from build123d import *

# Parameters (mm, degrees)
SALIENTE_EXTRUIR1_START                = 8
CROQUIS1_R                             = 10
SALIENTE_EXTRUIR1_DEPTH                = 258
CROQUIS2_R                             = 15
SALIENTE_EXTRUIR2_DEPTH                = 3
CORTAR_EXTRUIR1_REACH                  = 268.845
CORTAR_EXTRUIR1_END_RADIUS             = 10
CROQUIS3_R                             = 3.075
CORTAR_EXTRUIR1_DIRECTION_2_REACH      = 268.845
CORTAR_EXTRUIR1_DIRECTION_2_END_RADIUS = 10
CORTAR_EXTRUIR2_START                  = 10
CORTAR_EXTRUIR2_DEPTH                  = 3.5
TALADRO_ROSCADO_M61_D                  = 5
TALADRO_ROSCADO_M61_DEPTH              = 11.497848452
TALADRO_ROSCADO_M61_TIP                = 1.502151548
CORTAR_EXTRUIR3_START                  = 10
CORTAR_EXTRUIR3_DEPTH                  = 3.5
CORTAR_EXTRUIR4_START                  = 125.5
CROQUIS9_R                             = 10
CROQUIS9_R_2                           = 9.5
CORTAR_EXTRUIR4_DEPTH                  = 1.3
CORTAR_EXTRUIR5_START                  = 214.543146
CROQUIS10_R                            = 10
CROQUIS10_R_2                          = 9.5
CORTAR_EXTRUIR5_DEPTH                  = 1.3
CORTAR_EXTRUIR6_START                  = -8
CROQUIS11_R                            = 10
CROQUIS11_R_2                          = 9.5
CORTAR_EXTRUIR6_DEPTH                  = 1.3


with BuildPart() as part:
    # Croquis1 → Saliente-Extruir1 (new body)
    with BuildSketch(Plane(origin=(0, 0, 0), x_dir=(0, 0, -1), z_dir=(1, 0, 0)).offset(SALIENTE_EXTRUIR1_START)):
        Circle(CROQUIS1_R)
    extrude(amount=SALIENTE_EXTRUIR1_DEPTH)

    # Croquis2 → Saliente-Extruir2 (add)
    with BuildSketch(Plane.ZY.offset(-70.5)):
        Circle(CROQUIS2_R)
    extrude(amount=SALIENTE_EXTRUIR2_DEPTH)

    # Cortar-Extruir1: up to this cylinder (the profile starts inside it)
    cortar_extruir1_end = Plane(origin=(248.5, 0, 0), z_dir=(-1, 0, 0)) * Cylinder(CORTAR_EXTRUIR1_END_RADIUS, 558.69, mode=Mode.PRIVATE)
    # Croquis3 → Cortar-Extruir1 (cut, up to the surface)
    with BuildSketch(Plane.XY, mode=Mode.PRIVATE) as cortar_extruir1_sk1:
        with Locations((248.5, 0)):
            Circle(CROQUIS3_R)
    cortar_extruir1_tool1 = extrude(cortar_extruir1_sk1.sketch, amount=-CORTAR_EXTRUIR1_REACH, mode=Mode.PRIVATE) & cortar_extruir1_end
    add(cortar_extruir1_tool1.solids().sort_by_distance((248.5, 0, 0))[0], mode=Mode.SUBTRACT)

    # Cortar-Extruir1 direction 2: up to this cylinder (the profile starts inside it)
    cortar_extruir1_direction_2_end = Plane(origin=(248.5, 0, 0), z_dir=(-1, 0, 0)) * Cylinder(CORTAR_EXTRUIR1_DIRECTION_2_END_RADIUS, 558.69, mode=Mode.PRIVATE)
    # Croquis3 → Cortar-Extruir1 direction 2 (cut, up to the surface)
    with BuildSketch(Plane.XY, mode=Mode.PRIVATE) as cortar_extruir1_direction_2_sk1:
        with Locations((248.5, 0)):
            Circle(CROQUIS3_R)
    cortar_extruir1_direction_2_tool1 = extrude(cortar_extruir1_direction_2_sk1.sketch, amount=CORTAR_EXTRUIR1_DIRECTION_2_REACH, mode=Mode.PRIVATE) & cortar_extruir1_direction_2_end
    add(cortar_extruir1_direction_2_tool1.solids().sort_by_distance((248.5, 0, 0))[0], mode=Mode.SUBTRACT)

    # Croquis4 → Cortar-Extruir2 (cut)
    with BuildSketch(Plane(origin=(0, 0, 0), x_dir=(1, 0, 0), z_dir=(0, 1, 0)).offset(CORTAR_EXTRUIR2_START)):
        with BuildLine():
            Line((239, 3), (253, 3))
            ThreePointArc((253, 3), (256, 0), (253, -3))
            Line((253, -3), (239, -3))
            ThreePointArc((239, -3), (236, 0), (239, 3))
        make_face()
    extrude(amount=-CORTAR_EXTRUIR2_DEPTH, mode=Mode.SUBTRACT)

    # Taladro roscado M61
    with Locations(Plane(origin=(266, 0, 0), x_dir=(0, 0, 1), z_dir=(1, 0, 0))):
        with Locations((0, 0)):
            Hole(TALADRO_ROSCADO_M61_D / 2, depth=TALADRO_ROSCADO_M61_DEPTH)
            with Locations((0, 0, -(TALADRO_ROSCADO_M61_DEPTH + TALADRO_ROSCADO_M61_TIP / 2))):  # 118° drill point
                Cone(0, TALADRO_ROSCADO_M61_D / 2, TALADRO_ROSCADO_M61_TIP, mode=Mode.SUBTRACT)

    # Croquis8 → Cortar-Extruir3 (cut)
    with BuildSketch(Plane(origin=(0, 0, 0), x_dir=(1, 0, 0), z_dir=(0, 1, 0)).offset(CORTAR_EXTRUIR3_START)):
        with BuildLine():
            Line((78, 3), (112, 3))
            ThreePointArc((112, 3), (115, 0), (112, -3))
            Line((112, -3), (78, -3))
            ThreePointArc((78, -3), (75, 0), (78, 3))
        make_face()
    extrude(amount=-CORTAR_EXTRUIR3_DEPTH, mode=Mode.SUBTRACT)

    # Croquis9 → Cortar-Extruir4 (cut)
    with BuildSketch(Plane(origin=(0, 0, 0), x_dir=(0, 0, -1), z_dir=(1, 0, 0)).offset(CORTAR_EXTRUIR4_START)):
        with Locations(Location((0, 0, 0), (0, 0, 180))):
            Circle(CROQUIS9_R)
        Circle(CROQUIS9_R_2, mode=Mode.SUBTRACT)
    extrude(amount=CORTAR_EXTRUIR4_DEPTH, mode=Mode.SUBTRACT)

    # Croquis10 → Cortar-Extruir5 (cut)
    with BuildSketch(Plane(origin=(0, 0, 0), x_dir=(0, 0, -1), z_dir=(1, 0, 0)).offset(CORTAR_EXTRUIR5_START)):
        with Locations(Location((0, 0, 0), (0, 0, 180))):
            Circle(CROQUIS10_R)
        Circle(CROQUIS10_R_2, mode=Mode.SUBTRACT)
    extrude(amount=CORTAR_EXTRUIR5_DEPTH, mode=Mode.SUBTRACT)

    # Croquis11 → Cortar-Extruir6 (cut)
    with BuildSketch(Plane.ZY.offset(-8).offset(CORTAR_EXTRUIR6_START)):
        Circle(CROQUIS11_R)
        with Locations(Location((0, 0, 0), (0, 0, 180))):
            Circle(CROQUIS11_R_2, mode=Mode.SUBTRACT)
    extrude(amount=-CORTAR_EXTRUIR6_DEPTH, mode=Mode.SUBTRACT)


solid = part.part
Here's how the part is built. I have some questions about the finished solid (model axes, mm). A direction names the side the tool comes from. Round coordinates to 2 decimals unless told otherwise and drop trailing zeros. Loops run counter-clockwise (first coordinate to the right, second up) from the corner with the lowest first, then second, coordinate; pieces in that order, holes last. Notation, with made-up numbers: M 27.5,-34 L 85.5,-34 A33 ccw 85.5,-3 Z; hole C 74.5,-4.5 d7. An arc over 180 degrees is marked long. Write each question's results on one line, items separated by ' | '. Start each with the question number.
(1) On a 3-axis mill with a long thin cutter (end or side, diameter ignored), from which of +Z, -Z, +X, -X, +Y, -Y can I reach the whole of each face in a straight line? I mean faces 4 (the flat face through (95, 6.5, 0)), 5 (the flat face through (67.5, -10, 3)), 6 (the cylindrical face through (240.57, -8.872, -4.614)), 7 (the flat face through (126.8, 4, 9)). Say none if no direction works.
(2) I want a section at A-A (x = 248.5). Please give me the cut outline in (y, z) (3 decimals), then the cut area to 3 significant figures.
(3) Will these pins go through, and if not, where does the flat tip stop? P1, Ø2.5, axis at x = 98, y = 8, coming from the -Z side; P2, Ø0.9, axis at x = 247.5, y = 8, coming from the -Z side; P3, Ø0.9, axis at x = 93.5, y = 8.5, coming from the +Z side.
(4) Thinking about a two-plate mould opening in X: for faces 1 (the cylindrical face through (170.06, -9.76, 2.17)), 2 (the flat face through (246, 6.5, 0)), 3 (the conical face through (253, 0, 0)), which applies, pulls with the +X half, pulls with the -X half, needs draft (parallel to the pull), parting line crosses it, or undercut?
(5) I want a section at B-B (x = 123). Please give me the cut outline in (y, z).
(6) If I drill on probe 1 along Y at (x, z) = (257.75, 0); probe 2 along Y at (x, z) = (248.5, 3.25) (3 decimals); probe 3 along X at (y, z) = (0, -5) (3 decimals), over which ranges is the centre line in solid material (lowest first)? Write a range as from..to.
Solved:
1) face 4: +Y | face 5: -X | face 6: +X | face 7: none
2) outline: M -3.075,-9.515 L -3.075,9.515 A10 ccw Z; M 3.075,-9.515 A10 ccw 9.539,-3 L 6.5,-3 L 6.5,3 L 9.539,3 A10 ccw 3.075,9.515 Z | area: 173 mm²
3) P1: stops at z = -7.38 | P2: stops at z = -6.56 | P3: stops at z = 5.93
4) face 1: needs draft | face 2: undercut | face 3: pulls with the +X half
5) outline: C 0,0 d20
6) probe 1: y = -10..-2.5, 2.5..10 | probe 2: y = -9.457..-3.075, 3.075..9.457 | probe 3: x = 8..245.425, 251.575..266
